Can you work these out from the drawing? Everything is in mm from the part's minimum corner. Coordinates: 2 decimals unless noted, no trailing zeros. Write each loop counter-clockwise with the first axis right and the second up, starting at its lowest first coordinate (ties: lowest second). Pieces come first, ordered by that corner, then holes.
(1) Imagine slicing it at C-C, the plane x = 2.3. List the corners of the cut face in (y, z) for me (1 decimal).
(2) Imagine slicing it at A-A, the plane y = 7. List the corners of the cut face in (x, z) for me (1 decimal).
(3) For pin 1 Ø6 at (y, z) = (11.19, 59.17) entering from +X; pin 2 Ø1 at (x, y) = (2, 34.5) entering from +Z; pin 3 Ø1 at (x, y) = (1.5, 42.5) entering from +Z; pin 4 Ø1.5 at (x, y) = (3, 40.5) entering from +Z, each with a flat end and sliding along its axis, tell me the tip position at first contact or that it passes through.
(4) Thinking about a two-plate mould opening in Y: for the marked faces 1, 2 and 3, which applies, released by +Y, released by -Y, zero draft, split by the parting line, or undercut?
(5) Imagine slicing it at B-B, the plane z = 62.5. List the corners of the cut face in (x, y) for me (1 decimal).
(6) Imagine slicing it at D-D, the plane y = 13.5. List the corners of the cut face in (x, z) for me.
(7) Please list where these lines run through material, in increasing order: probe 1 along Z at (x, y) = (2.8, 53.5) (1 decimal); probe 2 along Y at (x, z) = (3.5, 63.5) (1 decimal); probe 3 along Y at (x, z) = (2.7, 12) (1 decimal).
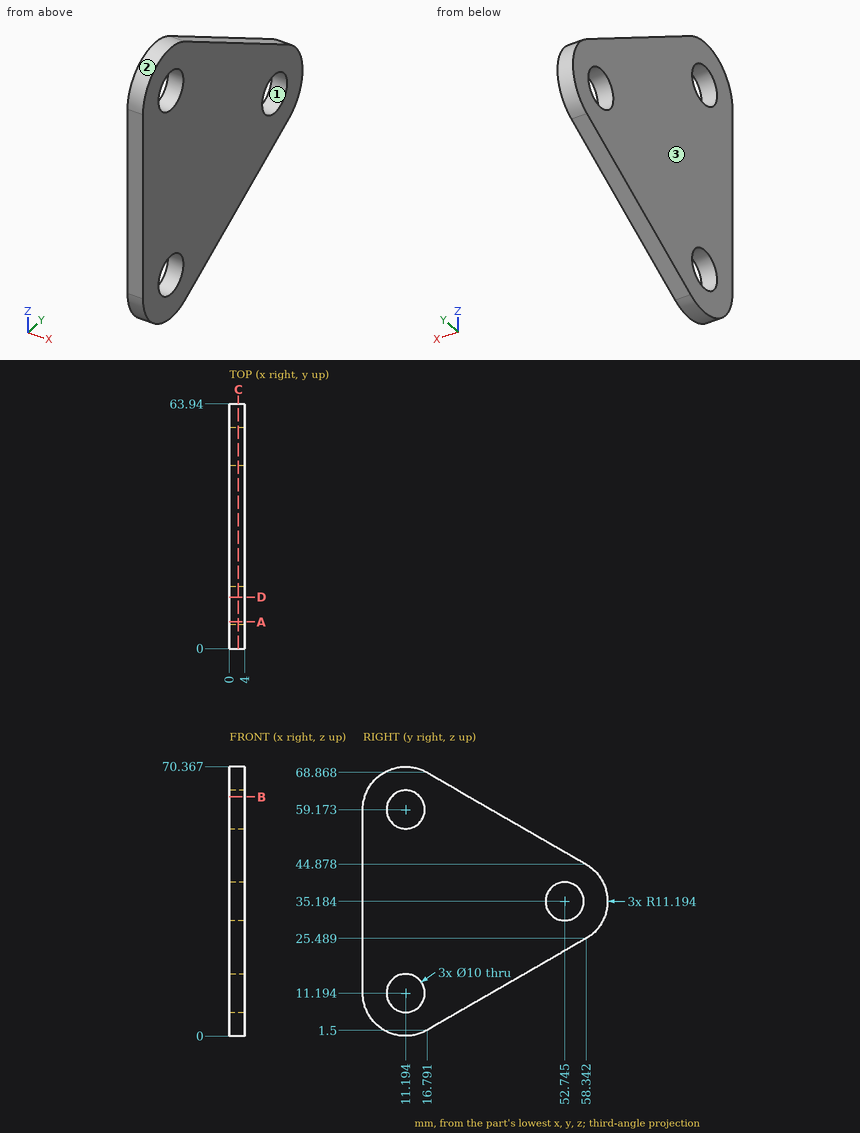
Recorded:
1. outline: (0, 11.2) arc R11.2 ccw to (16.8, 1.5) - (58.3, 25.5) arc R11.2 ccw to (58.3, 44.9) - (16.8, 68.9) arc R11.2 ccw to (0, 59.2) - close; hole circle Ø10 at (11.2, 11.2); hole circle Ø10 at (11.2, 59.2); hole circle Ø10 at (52.7, 35.2)
2. outline: (0, 0.8) - (4, 0.8) - (4, 8.5) - (0, 8.5) - close; (0, 13.9) - (4, 13.9) - (4, 56.5) - (0, 56.5) - close; (0, 61.9) - (4, 61.9) - (4, 69.6) - (0, 69.6) - close
3. pin 1: passes through
3. pin 2: stops at z = 58.93
3. pin 3: stops at z = 54.31
3. pin 4: stops at z = 55.61
4. face 1: undercut
4. face 2: split by the parting line
4. face 3: zero draft
5. outline: (0, 0.5) - (4, 0.5) - (4, 7.5) - (0, 7.5) - close; (0, 14.9) - (4, 14.9) - (4, 27.8) - (0, 27.8) - close
6. outline: (0, 0.24) - (4, 0.24) - (4, 6.76) - (0, 6.76) - close; (0, 15.63) - (4, 15.63) - (4, 54.74) - (0, 54.74) - close; (0, 63.61) - (4, 63.61) - (4, 70.13) - (0, 70.13) - close
7. probe 1: z = 22.7 to 30.2, 40.1 to 47.7
7. probe 2: y = 0.9 to 8.7, 13.7 to 26.1
7. probe 3: y = 0 to 6.3, 16.1 to 35
